For this review, take the finished solid that the model builds, in its own axes (mm). Face numbers are marked on the shaded views. A direction names the side the tool comes from. Round coordinates to 2 decimals unless told otherwise and drop trailing zeros. Write each loop counter-clockwise with the first axis right and the second up, starting at its lowest first coordinate (ties: lowest second). Pieces come first, ordered by that corner, then holes.
from build123d import *

# Parameters (mm, degrees)
F1_DEPTH = 9.652
F4_DEPTH = 45.72
F5_R     = 5.08
F6_R     = 5.518892
F7_W     = 10.16
F7_H     = 3
F8_DEPTH = 50.8


with BuildPart() as f1:
    # F0 (on Top) → F1 (new body)
    with BuildSketch(Plane.XY):
        Polygon((0, 13.647766), (0, 0), (0, -62.552234), (45.72, -62.552234), (45.72, 13.647766), align=None)
    extrude(amount=F1_DEPTH)

    # F3 (on Right) → F4 (join)
    with BuildSketch(Plane.YZ):
        Polygon((13.10063, -12), (13.10063, 0), (0.40063, 0), (0.40063, -6), (-17.37937, -6), (-17.37937, -12), align=None)
    extrude(amount=F4_DEPTH)

    # F5
    f5_edges = [f1.edges().sort_by_distance(p)[0] for p in [
        (45.72, 13.10063, -6),
        (0, 13.10063, -6),
    ]]
    fillet(f5_edges, radius=F5_R)

    # F6
    f6_edges = [f1.edges().sort_by_distance(p)[0] for p in [
        (45.72, 13.647766, 4.826),
        (0, 13.647766, 4.826),
    ]]
    fillet(f6_edges, radius=F6_R)

    # F7 (on face) → F8 (cut)
    with BuildSketch(Plane(origin=(0, 13.647766, 0), x_dir=(-1, 0, 0), z_dir=(0, 1, 0))):
        with Locations((-30.156892, 4.777829)):
            Rectangle(F7_W, F7_H)
        with Locations((-14.916892, 4.777829)):
            Rectangle(F7_W, F7_H)
    extrude(amount=-F8_DEPTH, mode=Mode.SUBTRACT)


solid = f1.part
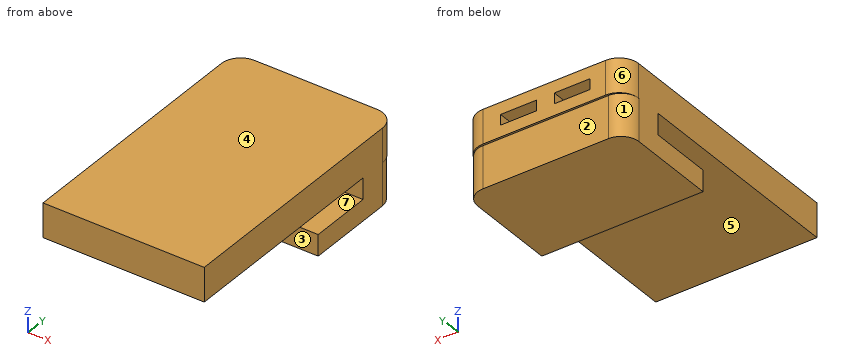
(1) For line 1 along Z through (x, y) = (19.5, -29); line 2 along Z through (x, y) = (39, -25.5); line 3 along Y through (x, z) = (20.5, -3.75), list the stretches that pass through material, from the lowest coordinate up.
Geometry check:
line 1: z = 0 to 3.28, 6.28 to 9.65
line 2: z = 0 to 9.65
line 3: y = 0.4 to 13.1
(2) We need section D-D, the plane z = -4. Give the boundary of the cut face in (x, y), and give its area (3 significant figures).
Geometry check:
outline: (0, 0.4) - (45.72, 0.4) - (45.72, 8.02) arc R5.08 ccw to (40.64, 13.1) - (5.08, 13.1) arc R5.08 ccw to (0, 8.02) - close
area: 570 mm2
(3) We need section A-A, the plane y = -4.5. Give the boundary of the cut face in (x, z).
Geometry check:
outline: (0, -12) - (45.72, -12) - (45.72, -6) - (0, -6) - close; (0, 0) - (45.72, 0) - (45.72, 9.65) - (0, 9.65) - close; hole (9.84, 3.28) - (20, 3.28) - (20, 6.28) - (9.84, 6.28) - close; hole (25.08, 3.28) - (35.24, 3.28) - (35.24, 6.28) - (25.08, 6.28) - close
(4) We need section C-C, the plane x = 16. Give the boundary of the cut face in (y, z).
Geometry check:
outline: (-62.55, 0) - (0.4, 0) - (0.4, -6) - (-17.38, -6) - (-17.38, -12) - (13.1, -12) - (13.1, 0) - (13.65, 0) - (13.65, 3.28) - (-37.15, 3.28) - (-37.15, 6.28) - (13.65, 6.28) - (13.65, 9.65) - (-62.55, 9.65) - close
(5) For pin 1 Ø3.5 at (x, z) = (28, -3.5) entering from +Y; pin 2 Ø8 at (x, z) = (34.5, -1) entering from -Y; pin 3 Ø3 at (x, y) = (29.5, -22.5) entering from -Z; pin 4 Ø1.8 at (x, z) = (28.5, -3) entering from -Y, all flat-tipped, find the tip position at first contact; note any pin that passes through.
Geometry check:
pin 1: stops at y = 13.1
pin 2: stops at y = -62.55
pin 3: stops at z = 0
pin 4: stops at y = 0.4
(6) We need section B-B, the plane y = -31. Give the boundary of the cut face in (x, z).
Geometry check:
outline: (0, 0) - (45.72, 0) - (45.72, 9.65) - (0, 9.65) - close; hole (9.84, 3.28) - (20, 3.28) - (20, 6.28) - (9.84, 6.28) - close; hole (25.08, 3.28) - (35.24, 3.28) - (35.24, 6.28) - (25.08, 6.28) - close
(7) Mouldability with a two-part tool opening along Z and no side actions: class the marked faces 4, 5, 6 and 7 as pulls with the +Z half, pulls with the -Z half, needs draft (parallel to the pull), parting line crosses it, or undercut.
Geometry check:
face 4: pulls with the +Z half
face 5: undercut
face 6: needs draft
face 7: undercut
(8) For the marked faces 1, 2 and 3, list the 3-axis set-ups (+Z, -Z, +X, -X, +Y, -Y) from which the entire face can be reached by the end or side of a thin tool; tool diameter is ignored.
Geometry check:
face 1: -Z, -X, +Y
face 2: -Z, +X, -X, +Y
face 3: -Z, +X, -X, -Y
